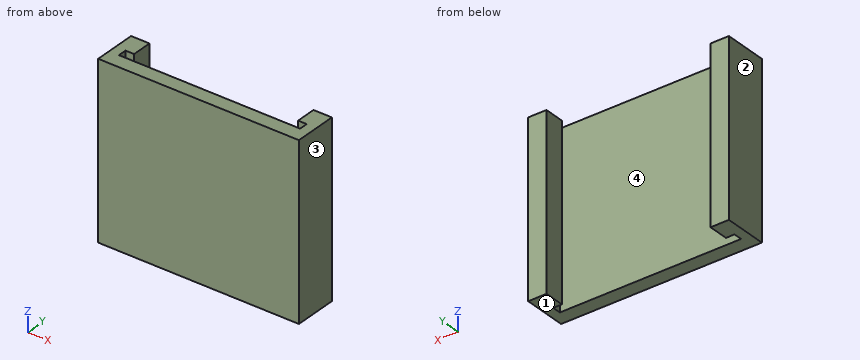
from build123d import *

# Parameters (mm, degrees)
SKETCH1_W           = 70
SKETCH1_H           = 60
BOSS_EXTRUDE1_DEPTH = 5
SKETCH2_W           = 3.4
SKETCH2_H           = 60
BOSS_EXTRUDE2_DEPTH = 10
SKETCH5_W           = 60
SKETCH5_H           = 7
BOSS_EXTRUDE5_DEPTH = 3
SKETCH6_W           = 60
SKETCH6_H           = 7
BOSS_EXTRUDE6_DEPTH = 3


with BuildPart() as part:
    # Sketch1 → Boss-Extrude1 (new body)
    with BuildSketch(Plane(origin=(0, 0, 0), x_dir=(1, 0, 0), z_dir=(0, 1, 0))):
        Rectangle(SKETCH1_W, SKETCH1_H)
    extrude(amount=BOSS_EXTRUDE1_DEPTH)

    # Sketch2 → Boss-Extrude2 (add)
    with BuildSketch(Plane(origin=(0, 5, 0), x_dir=(1, 0, 0), z_dir=(0, 1, 0))):
        with Locations((-33.3, 0)):
            Rectangle(SKETCH2_W, SKETCH2_H)
        with Locations((33.3, 0)):
            Rectangle(SKETCH2_W, SKETCH2_H)
    extrude(amount=BOSS_EXTRUDE2_DEPTH)

    # Sketch5 → Boss-Extrude5 (add)
    with BuildSketch(Plane(origin=(-31.6, 0, 0), x_dir=(0, 0, -1), z_dir=(1, 0, 0))):
        with Locations((0, 11.5)):
            Rectangle(SKETCH5_W, SKETCH5_H)
    extrude(amount=BOSS_EXTRUDE5_DEPTH)

    # Sketch6 → Boss-Extrude6 (add)
    with BuildSketch(Plane.ZY.offset(-31.6)):
        with Locations((0, 11.5)):
            Rectangle(SKETCH6_W, SKETCH6_H)
    extrude(amount=BOSS_EXTRUDE6_DEPTH)


solid = part.part
Read the model definition and answer for the solid it produces. Units are mm, in the model's axes. Face numbers are marked on the shaded views. Give positions to 0.01 mm unless a question says otherwise; leave off trailing zeros. Loops run counter-clockwise (first coordinate to the right, second up) from the corner with the lowest first, then second, coordinate; pieces in that order, holes last. Notation, with made-up numbers: M -16,88.5 L 41,88.5 A23 ccw 41,104.5 Z; hole C 14.5,-28 d4. An arc over 180 degrees is marked long. Write each question's results on one line, items separated by ' | '.
1. The mould has two halves that part along X. Classify the marked faces 1, 2, 3 and 4: pulls with the +X half, pulls with the -X half, needs draft (parallel to the pull), parting line crosses it, or undercut.
Values:
face 1: needs draft | face 2: pulls with the -X half | face 3: pulls with the +X half | face 4: undercut
2. Section B-B on z = -19.5 is taken. Give the vertices of the cut face in (x, y), plus the area to 3 significant figures.
Values:
outline: M -35,0 L 35,0 L 35,15 L 28.6,15 L 28.6,8 L 31.6,8 L 31.6,5 L -31.6,5 L -31.6,8 L -28.6,8 L -28.6,15 L -35,15 Z | area: 460 mm^2
3. Section C-C on y = 11.75 is taken. Give the vertices of the cut face in (x, z).
Values:
outline: M -35,-30 L -28.6,-30 L -28.6,30 L -35,30 Z; M 28.6,-30 L 35,-30 L 35,30 L 28.6,30 Z
4. Section A-A on y = 6 is taken. Give the vertices of the cut face in (x, z), plus the area to 3 significant figures.
Values:
outline: M -35,-30 L -31.6,-30 L -31.6,30 L -35,30 Z; M 31.6,-30 L 35,-30 L 35,30 L 31.6,30 Z | area: 408 mm^2
5. Straight lines are drawn through the part: line 1 (X direction, y = 5.5, z = 13); line 2 (X direction, y = 9, z = 19); line 3 (Y direction, x = 31.5, z = 20.5). For each, find the intervals that lie inside material, in ascending order. Write a range as [from, to].
Values:
line 1: x = [-35, -31.6], [31.6, 35] | line 2: x = [-35, -28.6], [28.6, 35] | line 3: y = [0, 5], [8, 15]
6. Section D-D on x = 16.5 is taken. Give the vertices of the cut face in (y, z), plus the area to 3 significant figures.
Values:
outline: M 0,-30 L 5,-30 L 5,30 L 0,30 Z | area: 300 mm^2
7. Given pin 1 (2.5 mm diameter, centred on x = 29.5, z = -11, fed in from -Y); pin 2 (18 mm diameter, centred on x = -11, z = -11.5, fed in from +Y), each flat-ended and moving along its own axis, determine where each tip first touches the part or whether it passes through.
Values:
pin 1: stops at y = 0 | pin 2: stops at y = 5
